from build123d import *

# Parameters (mm, degrees)
F1_DEPTH = 38
F3_DEPTH = 93
F5_DEPTH = 35
F6_R     = 20.15
F7_DEPTH = 26


with BuildPart() as f1:
    # F0 (on Top) → F1 (new body)
    with BuildSketch(Plane.XY):
        with BuildLine():
            Line((21.6, -7.9018985061), (21.6, 7.9018985061))
            ThreePointArc((21.6, 7.9018985061), (0, 23), (-21.6, 7.9018985061))
            Line((-21.6, 7.9018985061), (-21.6, -7.9018985061))
            ThreePointArc((-21.6, -7.9018985061), (0, -23), (21.6, -7.9018985061))
        make_face()
    extrude(amount=F1_DEPTH)

    # F2 (on face) → F3 (join)
    with BuildSketch(Plane.XY.offset(38)):
        with BuildLine():
            Line((11.5, 0), (11.5, 15.748015748))
            ThreePointArc((11.5, 15.748015748), (0, 19.5), (-11.5, 15.748015748))
            Line((-11.5, 15.748015748), (-11.5, -15.748015748))
            ThreePointArc((-11.5, -15.748015748), (0, -19.5), (11.5, -15.748015748))
            Line((11.5, -15.748015748), (11.5, 0))
        make_face()
    extrude(amount=F3_DEPTH)

    # F4 (on face) → F5 (cut)
    with BuildSketch(Plane.YZ.offset(11.5)):
        with BuildLine():
            ThreePointArc((15.748015748, 120.2564661625), (18.8743223664, 114.4792683229), (19.9554745068, 108))
            Line((19.9554745068, 108), (37.2544378042, 135.0286304951))
            Line((37.2544378042, 135.0286304951), (-38.2512100041, 135.0286304951))
            Line((-38.2512100041, 135.0286304951), (-19.9554745068, 108))
            ThreePointArc((-19.9554745068, 108), (-18.8743223664, 114.4792683229), (-15.748015748, 120.2564661625))
            Line((-15.748015748, 120.2564661625), (-15.748015748, 131))
            Line((-15.748015748, 131), (15.748015748, 131))
            Line((15.748015748, 131), (15.748015748, 120.2564661625))
        make_face()
        with BuildLine():
            ThreePointArc((-15.748015748, 120.2564661625), (0, 127.9554745068), (15.748015748, 120.2564661625))
            Line((15.748015748, 120.2564661625), (15.748015748, 131))
            Line((15.748015748, 131), (-15.748015748, 131))
            Line((-15.748015748, 131), (-15.748015748, 120.2564661625))
        make_face()
    extrude(amount=-F5_DEPTH, mode=Mode.SUBTRACT)

    # F6 (on face) → F7 (cut)
    with BuildSketch(Plane(origin=(0, 0, 0), x_dir=(1, 0, 0), z_dir=(0, 0, -1))):
        Circle(F6_R)
    extrude(amount=-F7_DEPTH, mode=Mode.SUBTRACT)


solid = f1.part
For this review, take the finished solid that the model builds, in its own axes (mm). A direction names the side the tool comes from. Round coordinates to 2 decimals unless told otherwise and drop trailing zeros. Write each loop counter-clockwise with the first axis right and the second up, starting at its lowest first coordinate (ties: lowest second). Pieces come first, ordered by that corner, then holes. Notation, with made-up numbers: (-18.5, -25) -> (35.5, -25) arc R16 cw to (35.5, -7) -> close; hole circle Ø9 at (7, 47). An arc over 180 degrees is marked (long way). Put each result on its own line as item: value.
Q1. Consider section C-C on y = 0. State the section outline as (x, z) points, and give its area (3 significant figures).
Determined:
outline: (-21.6, 0) -> (-20.15, 0) -> (-20.15, 26) -> (20.15, 26) -> (20.15, 0) -> (21.6, 0) -> (21.6, 38) -> (11.5, 38) -> (11.5, 127.96) -> (-11.5, 127.96) -> (-11.5, 38) -> (-21.6, 38) -> close
area: 2,660 mm^2
Q2. Consider section D-D on y = 13.5. State the section outline as (x, z) points.
Determined:
outline: (-18.62, 0) -> (-14.96, 0) -> (-14.96, 26) -> (14.96, 26) -> (14.96, 0) -> (18.62, 0) -> (18.62, 38) -> (11.5, 38) -> (11.5, 122.7) -> (-11.5, 122.7) -> (-11.5, 38) -> (-18.62, 38) -> close
Q3. To check wall thickness, follow L1, parallel to Y at x = 0, z = 5.5; L2, parallel to X at y = 0, z = 7; L3, parallel to Z at x = 18, y = 12. State the ranges of each line that lie inside material, in increasing order. Write a range as [from, to].
Determined:
L1: y = [-23, -20.15], [20.15, 23]
L2: x = [-21.6, -20.15], [20.15, 21.6]
L3: z = [0, 38]
Q4. Clearance check with flat-ended pins moving along their axes: pin 1 Ø9.5 at (y, z) = (4.5, 70.5) entering from +X; pin 2 Ø6 at (x, z) = (-14, 79) entering from -Y; pin 3 Ø1.5 at (x, z) = (-3.5, 104) entering from +Y. State where each tip first meets the part, or that it passes through.
Determined:
pin 1: stops at x = 11.5
pin 2: stops at y = -16.1
pin 3: stops at y = 19.31
Q5. Consider section B-B on x = 0. State the section outline as (y, z) points, and give its area (3 significant figures).
Determined:
outline: (-23, 0) -> (-20.15, 0) -> (-20.15, 26) -> (20.15, 26) -> (20.15, 0) -> (23, 0) -> (23, 38) -> (19.5, 38) -> (19.5, 112.24) arc R19.96 ccw to (-19.5, 112.24) -> (-19.5, 38) -> (-23, 38) -> close
area: 4,050 mm^2
Q6. The part is to be moulded in two halves that separate along Y. For faces 1 (the flat face through (14, 0, 38)), 2 (the flat face through (0, 0, 26)), 3 (the cylindrical face through (0, -23, 19)), say which applies: released by +Y, released by -Y, zero draft, split by the parting line, or undercut.
Determined:
face 1: zero draft
face 2: undercut
face 3: released by -Y
Q7. Machinability: for faces 4 (the cylindrical face through (0.2, 19.5, 78.6)), 5 (the flat face through (11.5, 0, 82)), 6 (the cylindrical face through (18.613, 7.718, 12.818)), 7 (the cylindrical face through (-0.2, -19.5, 78.6)), which of the approach directions +Z, -Z, +X, -X, +Y, -Y give a long, thin tool a straight path to every point of the face, cutting with its end or side? Answer none if there is none.
Determined:
face 4: +Z, +Y
face 5: +Z, +X, +Y, -Y
face 6: -Z
face 7: +Z, -Y
Q8. Consider section A-A on z = 9. State the section outline as (x, y) points.
Determined:
outline: (-21.6, -7.9) arc R23 ccw to (21.6, -7.9) -> (21.6, 7.9) arc R23 ccw to (-21.6, 7.9) -> close; hole circle Ø40.3 at (0, 0)
